Autodesk Inventor part; units mm, degrees
ref_plane "YZ Plane" through (0, 0, 0) normal (1, 0, 0) x (0, 1, 0)
ref_plane "XZ Plane" through (0, 0, 0) normal (0, 1, 0) x (-1, 0, 0)
ref_plane "XY Plane" through (0, 0, 0) normal (0, 0, 1) x (1, 0, 0)
sketch "스케치1" plane through (0, 0, 0) normal (0, 0, 1) x (1, 0, 0)
  line L0 (-67.5, 0) -> (67.5, 0) construction
  line L1 (-67.5, -10) -> (67.5, -10)
  line L2 (67.5, 10) -> (-67.5, 10)
  arc A0 (-67.5, 10) -> (-67.5, -10) centre (-67.5, 0) ccw
  arc A1 (67.5, -10) -> (67.5, 10) centre (67.5, 0) ccw
  circle A2 centre (-67.5, 0) radius 5
  circle A3 centre (67.5, 0) radius 5
  circle A4 centre (27.5, 0) radius 5
  point P0 (0, 0)
  dimension "d1" = 20
  dimension "d2" = 10
  dimension "d3" = 10
  dimension "d7" = 10
  dimension "d8" = 40
  dimension "d9" = 95
extrude "돌출1" add sketch "스케치1" along normal blind 5
properties part number "link_l1"
Verification items for the finished model (mm, model axes). Give positions to 0.01 mm unless a question says otherwise; leave off trailing zeros. Order: outer loops, then holes, each group sorted by start corner. A loop starts at its lowest first (then second) coordinate and runs counter-clockwise, first axis right, second up. Notation, with made-up numbers: (52.25, 65) -> (72.25, 65) arc R18 ccw to (72.25, 84) -> close; hole circle Ø3 at (68.5, -29). An arc over 180 degrees is marked (long way). One line per item, written item: value.
(1) Gauge pin test, flat ends, axial feed: pin 1 (2 mm diameter, centred on y = 7.5, z = 0.5, fed in from -X); pin 2 (6 mm diameter, centred on x = 27.5, y = 0, fed in from -Z). Record the tip position at first contact, or that the pin passes through.
Final values:
pin 1: x = -75.1
pin 2: through
(2) Sectioned sample at A-A on z = 2.05. Record the cut outline in (x, y).
Final values:
outline: (-67.5, -10) -> (67.5, -10) arc R10 ccw to (67.5, 10) -> (-67.5, 10) arc R10 ccw to start; hole circle Ø10 at (-67.5, 0); hole circle Ø10 at (27.5, 0); hole circle Ø10 at (67.5, 0)
(3) Sectioned sample at D-D on y = 8. Record the cut outline in (x, z).
Final values:
outline: (-73.5, 0) -> (73.5, 0) -> (73.5, 5) -> (-73.5, 5) -> close
(4) Scan lines: line 1 along Y through (x, z) = (-67.5, 3.45); line 2 along X through (y, z) = (1.5, 4.75); line 3 along X through (y, z) = (-4, 1.85). Record each from-to range of solid material in increasing order. Write a range as [from, to].
Final values:
line 1: [-10, -5], [5, 10]
line 2: [-77.39, -72.27], [-62.73, 22.73], [32.27, 62.73], [72.27, 77.39]
line 3: [-76.67, -70.5], [-64.5, 24.5], [30.5, 64.5], [70.5, 76.67]
(5) Draft check along X on faces 1 (the face through (-77.5, -0.2, 2.5)), 2 (the face through (1, 10, 2)), 3 (the face through (22.505, -0.22, 2.465)). Enter one of: pulls with the +X half, pulls with the -X half, needs draft (parallel to the pull), parting line crosses it, or undercut.
Final values:
face 1: pulls with the -X half
face 2: needs draft
face 3: undercut
(6) Sectioned sample at B-B on y = -1.5. Record the cut outline in (x, z).
Final values:
outline: (-77.39, 0) -> (-72.27, 0) -> (-72.27, 5) -> (-77.39, 5) -> close; (-62.73, 0) -> (22.73, 0) -> (22.73, 5) -> (-62.73, 5) -> close; (32.27, 0) -> (62.73, 0) -> (62.73, 5) -> (32.27, 5) -> close; (72.27, 0) -> (77.39, 0) -> (77.39, 5) -> (72.27, 5) -> close
(7) Sectioned sample at C-C on x = 27.5. Record the cut outline in (y, z), then the cut area to 3 significant figures.
Final values:
outline: (-10, 0) -> (-5, 0) -> (-5, 5) -> (-10, 5) -> close; (5, 0) -> (10, 0) -> (10, 5) -> (5, 5) -> close
area: 50.0 mm^2
